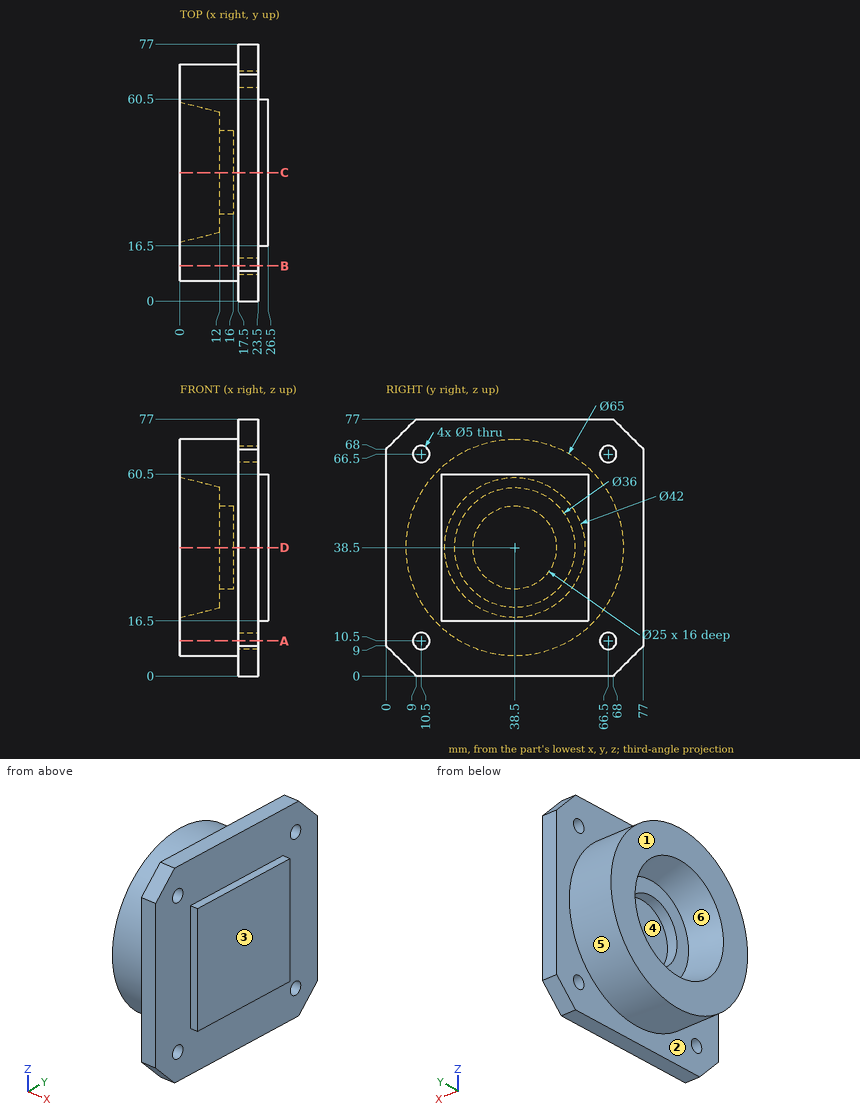
Design review of the part shown in the three views and the two pictorial views. Dimensions are in mm from the part's minimum x, y and z. A direction names the side the tool comes from. Give positions to 0.01 mm unless a question says otherwise; leave off trailing zeros. Loops run counter-clockwise (first coordinate to the right, second up) from the corner with the lowest first, then second, coordinate; pieces in that order, holes last. Notation, with made-up numbers: (-33, -39.5) -> (-12, -39.5) arc R19 cw to (-12, -4.5) -> close; hole circle Ø5 at (85.5, -6.75). An arc over 180 degrees is marked (long way). Put each result on its own line as item: value. Start each with the question number.
1. We need section C-C on y = 38.5. State the section outline as (x, z) points, then the cut area to 3 significant figures.
2. For the marked faces 1 and 2, list the 3-axis set-ups (+Z, -Z, +X, -X, +Y, -Y) from which the entire face can be reached by the end or side of a thin tool; tool diameter is ignored.
3. Wall thickness on probe 1 along Y at (x, z) = (21.9, 10.5); probe 2 along Y at (x, z) = (14.5, 38.5); probe 3 along X at (y, z) = (5.5, 16.5): over which ranges is each line inside the solid? List them lowest first.
4. We need section A-A on z = 10.5. State the section outline as (x, y) points.
5. Clearance check with flat-ended pins moving along their axes: P1, Ø20, axis at y = 38.5, z = 38.5, coming from the -X side; P2, Ø3.5, axis at x = 25.5, y = 34, coming from the -Z side; P3, Ø12, axis at x = 10.5, y = 58.5, coming from the -Z side. State where each tip first meets the part, or that it passes through.
6. Mouldability with a two-part tool opening along Y and no side actions: class the marked faces 3, 4, 5 and 6 as released by +Y, released by -Y, zero draft, split by the parting line, or undercut.
Determined:
1. outline: (0, 6) -> (17.5, 6) -> (17.5, 0) -> (23.5, 0) -> (23.5, 16.5) -> (26.5, 16.5) -> (26.5, 60.5) -> (23.5, 60.5) -> (23.5, 77) -> (17.5, 77) -> (17.5, 71) -> (0, 71) -> (0, 59.5) -> (12, 56.5) -> (12, 51) -> (16, 51) -> (16, 26) -> (12, 26) -> (12, 20.5) -> (0, 17.5) -> close
1. area: 1,160 mm^2
2. face 1: +Z, -Z, -X, +Y, -Y
2. face 2: -X
3. probe 1: 0 to 8, 13 to 64, 69 to 77
3. probe 2: 6 to 26, 51 to 71
3. probe 3: 17.5 to 23.5
4. outline: (0, 22) -> (17.5, 22) -> (17.5, 13) -> (23.5, 13) -> (23.5, 64) -> (17.5, 64) -> (17.5, 55) -> (0, 55) -> close; (17.5, 0) -> (23.5, 0) -> (23.5, 8) -> (17.5, 8) -> close; (17.5, 69) -> (23.5, 69) -> (23.5, 77) -> (17.5, 77) -> close
5. P1: x = 16
5. P2: z = 16.5
5. P3: z = 9.17
6. face 3: zero draft
6. face 4: undercut
6. face 5: split by the parting line
6. face 6: undercut
